Autodesk Inventor part; units mm, degrees
ref_plane "YZ Plane" through (0, 0, 0) normal (1, 0, 0) x (0, 1, 0)
ref_plane "XZ Plane" through (0, 0, 0) normal (0, 1, 0) x (-1, 0, 0)
ref_plane "XY Plane" through (0, 0, 0) normal (0, 0, 1) x (1, 0, 0)
sketch "Sketch1" plane through (0, 0, 0) normal (0, 0, 1) x (1, 0, 0)
  circle A0 centre (0, 0) radius 16.002 construction
  line L0 (8.2843, 20) -> (20, 8.2843)
  line L1 (20, 8.2843) -> (20, -8.2843)
  line L2 (20, -8.2843) -> (8.2843, -20)
  line L3 (8.2843, -20) -> (-8.2843, -20)
  line L4 (-8.2843, -20) -> (-20, -8.2843)
  line L5 (-20, -8.2843) -> (-20, 8.2843)
  line L6 (-20, 8.2843) -> (-8.2843, 20)
  line L7 (-8.2843, 20) -> (8.2843, 20)
  dimension "d0" = 32.004
  dimension "d2" = 40
extrude "Extrusion1" add sketch "Sketch1" along normal blind 30
chamfer "Chamfer1" distance 5 angle 45 8 edges at (-14.1421, 14.1421, 0) (-20, 0, 0) (-14.1421, -14.1421, 0) (0, -20, 0) (14.1421, -14.1421, 0) (20, 0, 0) (14.1421, 14.1421, 0) (0, 20, 0)
sketch "Sketch2" plane through (0, 0, 0) normal (0, 0, -1) x (-1, 0, 0)
  circle A0 centre (0, 0) radius 16.002 construction
  circle A1 centre (0, 0) radius 16.302
  dimension "d8" = 32.004
  dimension "d9" = 0.3
extrude "Extrusion2" cut sketch "Sketch2" against normal blind 8
sketch "Sketch4" plane through (0, 0, 30) normal (0, 0, 1) x (1, 0, 0)
  line L0 (-7.5, -7.5) -> (7.5, -7.5)
  line L1 (7.5, -7.5) -> (7.5, 7.5)
  line L2 (7.5, 7.5) -> (-7.5, 7.5)
  line L3 (-7.5, 7.5) -> (-7.5, -7.5)
  line L4 (-7.5, -7.5) -> (7.5, 7.5) construction
  line L5 (7.5, -7.5) -> (-7.5, 7.5) construction
  point P0 (0, 0)
  dimension "d18" = 15
  dimension "d19" = 15
extrude "Extrusion4" cut sketch "Sketch4" against normal blind 5
sketch "Sketch3" plane through (-8.2843, -20, 30) normal (-0.7071, -0.7071, 0) x (-0.7071, 0.7071, 0)
  line L0 (12.2843, 11) -> (4.2843, 11) construction
  line L1 (4.2843, 11) -> (4.2843, 23) construction
  line L2 (4.2843, 23) -> (12.2843, 23) construction
  line L3 (12.2843, 23) -> (12.2843, 11) construction
  line L4 (12.2843, 11) -> (4.2843, 23) construction
  line L5 (4.2843, 11) -> (12.2843, 23) construction
  line L6 (8.2843, 17) -> (8.2843, 30) construction
  circle A0 centre (8.2843, 11) radius 1.15
  circle A1 centre (12.2843, 23) radius 1.15
  circle A2 centre (4.2843, 23) radius 1.15
  dimension "d12" = 13
  dimension "d13" = 12
  dimension "d14" = 8
  dimension "d15" = 2.3
extrude "Extrusion3" cut sketch "Sketch3" against normal blind 3
pattern_circular "Circular Pattern1" count 4 over 360 about axis through (0, 0, -10) along (0, 0, 1) of "Extrusion3"
Input: part model. Units: mm. Frame: model coordinates. A direction names the side the tool comes from. Coordinates: 2 decimals unless noted, no trailing zeros. Order: outer loops, then holes, each group sorted by start corner. A loop starts at its lowest first (then second) coordinate and runs counter-clockwise, first axis right, second up. Notation, with made-up numbers: M 61,50.25 L 111,50.25 A24 ccw 111,62.25 Z; hole C -36,74 d9. An arc over 180 degrees is marked long. Answer as CSV lines item,"result".
1. Section A-A (z = 3.5). Return the cut outline in (x, y).
Reported:
outline,"M -18.5,-7.66 L -7.66,-18.5 L 7.66,-18.5 L 18.5,-7.66 L 18.5,7.66 L 7.66,18.5 L -7.66,18.5 L -18.5,7.66 Z; hole C 0,0 d32.6"
2. Section D-D (y = 5). Return the cut outline in (x, z).
Reported:
outline,"M -20,5 L -15.52,0.52 L -15.52,8 L 15.52,8 L 15.52,0.52 L 20,5 L 20,30 L 7.5,30 L 7.5,25 L -7.5,25 L -7.5,30 L -20,30 Z"
3. Material intervals for line 1 (Y direction, x = 9.5, z = 7.25); line 2 (X direction, y = 0, z = 6); line 3 (X direction, y = -9, z = 7), sorted ascending. Write a range as from..to.
Reported:
line 1,"-18.78..-16.74, -14.54..-13.25, 13.25..14.54, 16.74..18.78"
line 2,"-20..-16.3, 16.3..20"
line 3,"-19.28..-16.28, -15.04..-13.59, 13.59..15.04, 16.28..19.28"
4. Access query for faces 5 (the flat face through (-9.2, 14.84, 6.98)), 6 (the flat face through (0, -20, 17)), 7 (the flat face through (0, 0, 8)), 8 (the flat face through (-20, 0, 17)), 9 (the flat face through (0, 0, 25)). Directions: +Z, -Z, +X, -X, +Y, -Y. A direction counts if a zero-diameter tool reaches every point of the face in a straight line with its end or side. Return the directions, or none.
Reported:
face 5,"none"
face 6,"+Z, -Z, +X, -X, -Y"
face 7,"-Z"
face 8,"+Z, -Z, -X, +Y, -Y"
face 9,"+Z"
5. First-contact query: P1, Ø4, axis at x = -13, y = -12.5, coming from the -Z side; P2, Ø1.5, axis at x = 16, z = 16, coming from the +Y side; P3, Ø5, axis at x = -10, z = 9, coming from the +Y side; P4, Ø7.5, axis at x = 3.5, y = -2.5, coming from the +Z side. Flat tips, straight axial feed; report the tip coordinate or a pass-through.
Reported:
P1,"z = 1.25"
P2,"y = 13.03"
P3,"y = 20"
P4,"z = 25"
6. Section B-B (z = 22.75). Return the cut outline in (x, y).
Reported:
outline,"M -20,-8.28 L -8.28,-20 L 8.28,-20 L 20,-8.28 L 20,8.28 L 8.28,20 L -8.28,20 L -20,8.28 Z"
7. Pull-direction query (X, two-part tool) for faces 1 (the flat face through (-12.678, 12.842, 3.045)), 2 (the flat face through (12.678, -12.842, 3.045)), 3 (the flat face through (0, 20, 17)), 4 (the cylindrical face through (-13.272, 12.919, 20.123)); classes: released by +X, released by -X, zero draft, split by the parting line, or undercut.
Reported:
face 1,"released by -X"
face 2,"released by +X"
face 3,"zero draft"
face 4,"undercut"
8. Section C-C (x = 0). Return the cut outline in (y, z), then the cut area to 3 significant figures.
Reported:
outline,"M -20,5 L -16.3,1.3 L -16.3,8 L 16.3,8 L 16.3,1.3 L 20,5 L 20,30 L 7.5,30 L 7.5,25 L -7.5,25 L -7.5,30 L -20,30 Z"
area,"841 mm2"
